Input: part model. Units: mm. Frame: model coordinates. A direction names the side the tool comes from. Give positions to 0.01 mm unless a question says otherwise; leave off trailing zeros. Loops run counter-clockwise (first coordinate to the right, second up) from the corner with the lowest first, then second, coordinate; pieces in that order, holes last. Notation, with made-up numbers: M 87.25,54.5 L 110.25,54.5 A22 cw 110.25,90.5 Z; hole C -36,53.25 d9. An arc over 180 degrees is marked long. Answer as a JSON object with one key per item and string values. Group by question number.
1) First-contact query: P1, Ø3.5, axis at y = 10, z = 1.5, coming from the -X side; P2, Ø12, axis at x = -137.5, y = 5.5, coming from the -Z side; P3, Ø5, axis at y = 11, z = 12.5, coming from the -X side. Flat tips, straight axial feed; report the tip coordinate or a pass-through.
2) Draft query along X for faces 1 (the flat face through (-124, 0, 0)), 2 (the flat face through (-144.62, 9.92, 10.7)), 3 (the flat face through (-85.14, 9.916, -14.703)), 4 (the cylindrical face through (-163.85, 17.97, -2.7)). Return one class per face: +X half, -X half, draft (parallel to the pull), parting line (faces both ways), or undercut.
3) Section query B-B on x = -160.9. Return loops of the section in (y, z), plus the area to 3 significant figures.
4) Section query A-A on z = 0. Return loops of the section in (x, y).
5) Section query C-C on y = 9.5. Return loops of the section in (x, z), plus the area to 3 significant figures.
6) Ray query, L1, parallel to X at y = 18.65, z = 0; L2, parallel to Z at x = -82.8, y = 17.35; L3, parallel to Y at x = -160, z = 8. Return the intervals inside material, ascending.
7) Section query D-D on x = -123. Return loops of the section in (y, z), plus the area to 3 significant figures.
8) Access query for faces 5 (the flat face through (-85, 4, 0)), 6 (the flat face through (-144.622, 9.916, -10.737)), 7 (the cylindrical face through (-80.8, 2, 5.9)). Directions: +Z, -Z, +X, -X, +Y, -Y. A direction counts if a zero-diameter tool reaches every point of the face in a straight line with its end or side. Return the directions, or none.
from build123d import *

# Parameters (mm, degrees)
SKETCH1_R           = 4
BOSS_EXTRUDE1_DEPTH = 4
SKETCH2_R           = 4
BOSS_EXTRUDE2_DEPTH = 4
BOSS_EXTRUDE5_DEPTH = 12
SKETCH6_R           = 2
CUT_EXTRUDE1_DEPTH  = 21
BOSS_EXTRUDE6_DEPTH = 12


with BuildPart() as part:
    # Sketch1 → Boss-Extrude1 (new body)
    with BuildSketch(Plane(origin=(0, 0, 0), x_dir=(1, 0, 0), z_dir=(0, 1, 0))):
        with BuildLine():
            Line((-75, 18.10605947), (-161.821193893, 10.459512504))
            ThreePointArc((-161.821193893, 10.459512504), (-171.4, 0), (-161.821193893, -10.459512504))
            Line((-161.821193893, -10.459512504), (-75, -18.10605947))
            Line((-75, -18.10605947), (-75, 18.10605947))
        make_face()
        with Locations((-160.9, 0)):
            Circle(SKETCH1_R, mode=Mode.SUBTRACT)
    extrude(amount=BOSS_EXTRUDE1_DEPTH)



with BuildPart() as body_2:
    # Sketch2 → Boss-Extrude2 (new body)
    with BuildSketch(Plane(origin=(0, 16, 0), x_dir=(1, 0, 0), z_dir=(0, 1, 0))):
        with BuildLine():
            Line((-75, 18.10605947), (-161.821193893, 10.459512504))
            ThreePointArc((-161.821193893, 10.459512504), (-171.4, 0), (-161.821193893, -10.459512504))
            Line((-161.821193893, -10.459512504), (-75, -18.10605947))
            Line((-75, -18.10605947), (-75, 18.10605947))
        make_face()
        with Locations((-160.9, 0)):
            Circle(SKETCH2_R, mode=Mode.SUBTRACT)
    extrude(amount=BOSS_EXTRUDE2_DEPTH)


with BuildPart() as part_1:
    add(part.part)

    add(body_2.part)  # Boss-Extrude5 merges body 2
    # Sketch5 → Boss-Extrude5 (add)
    with BuildSketch(Plane(origin=(0, 4, 0), x_dir=(1, 0, 0), z_dir=(0, 1, 0))):
        Polygon((-75, -18.10605947), (-75, -15.596382275), (-144.510751478, -9.47440673), (-144.730083357, -11.964766849), align=None)
        Polygon((-75, 15.596382275), (-75, 18.10605947), (-144.730083357, 11.964766849), (-144.510751478, 9.47440673), align=None)
    extrude(amount=BOSS_EXTRUDE5_DEPTH)

    # Sketch6 → Cut-Extrude1 (cut, through all)
    with BuildSketch(Plane(origin=(0, 0, 0), x_dir=(-1, 0, 0), z_dir=(0, -1, 0))):
        with Locations((82.8, -5.982385529)):
            Circle(SKETCH6_R)
        with Locations((82.8, 6.017614471)):
            Circle(SKETCH6_R)
    extrude(amount=-CUT_EXTRUDE1_DEPTH, mode=Mode.SUBTRACT)

    # Sketch7 → Boss-Extrude6 (add)
    with BuildSketch(Plane(origin=(0, 4, 0), x_dir=(1, 0, 0), z_dir=(0, 1, 0))):
        Polygon((-144.510751478, 9.47440673), (-144.510751478, -9.47440673), (-95, -13.834935185), (-95, 13.834935185), align=None)
    extrude(amount=BOSS_EXTRUDE6_DEPTH)


solid = part_1.part
Output:
{
 "1": {"P1": "stops at x = -144.51", "P2": "stops at z = -13.13", "P3": "stops at x = -144.73"},
 "2": {"face 1": "draft", "face 2": "-X half", "face 3": "+X half", "face 4": "undercut"},
 "3": {"outline": "M 0,-10.54 L 4,-10.54 L 4,-4 L 0,-4 Z; M 0,4 L 4,4 L 4,10.54 L 0,10.54 Z; M 16,-10.54 L 20,-10.54 L 20,-4 L 16,-4 Z; M 16,4 L 20,4 L 20,10.54 L 16,10.54 Z", "area": "105 mm^2"},
 "4": {"outline": "M -171.4,0 L -164.9,0 L -164.9,4 L -171.4,4 Z; M -171.4,16 L -164.9,16 L -164.9,20 L -171.4,20 Z; M -156.9,0 L -75,0 L -75,4 L -95,4 L -95,16 L -75,16 L -75,20 L -156.9,20 L -156.9,16 L -144.51,16 L -144.51,4 L -156.9,4 Z"},
 "5": {"outline": "M -144.73,-11.96 L -75,-18.11 L -75,-15.6 L -95,-13.83 L -95,13.83 L -75,15.6 L -75,18.11 L -144.73,11.96 L -144.51,9.47 L -144.51,-9.47 Z", "area": "1,500 mm^2"},
 "6": {"L1": "x = -171.4 to -164.9, -156.9 to -75", "L2": "z = -17.42 to -8.02, -4.02 to 3.98, 7.98 to 17.42", "L3": "y = 0 to 4, 16 to 20"},
 "7": {"outline": "M 0,-13.88 L 20,-13.88 L 20,13.88 L 0,13.88 Z", "area": "555 mm^2"},
 "8": {"face 5": "+X", "face 6": "-X", "face 7": "+Y, -Y"}
}
